from build123d import *

# Parameters (mm, degrees)
F0_W      = 72
F0_H      = 72
F1_DEPTH  = 1.55
F2_W      = 9
F2_H      = 9
F3_DEPTH  = 1.551
F4_R      = 4
F5_W      = 21
F5_H      = 31
F6_DEPTH  = 4
F7_W      = 5.2
F7_H      = 8
F7_W_2    = 0.8
F8_DEPTH  = 2.5
F9_W      = 12.8
F9_H      = 38
F10_DEPTH = 5
F11_W     = 5.5
F11_H     = 11.5
F12_DEPTH = 2.5
F13_R     = 0.75
F14_DEPTH = 4.051
F15_W     = 4.5
F15_H     = 4.5
F16_DEPTH = 3
F17_W     = 7.4
F17_H     = 2.4
F18_DEPTH = 9.3


with BuildPart() as f1:
    # F0 (on Top) → F1 (new body)
    with BuildSketch(Plane.XY):
        with Locations((-36, -36)):
            Rectangle(F0_W, F0_H)
    extrude(amount=-F1_DEPTH)

    # F2 (on face) → F3 (cut, through all)
    with BuildSketch(Plane.XY):
        with Locations((-67.5, -67.5)):
            Rectangle(F2_W, F2_H)
        with Locations((-67.5, -4.5)):
            Rectangle(F2_W, F2_H)
        with Locations((-4.5, -4.5)):
            Rectangle(F2_W, F2_H)
        with Locations((-4.5, -67.5)):
            Rectangle(F2_W, F2_H)
    extrude(amount=-F3_DEPTH, mode=Mode.SUBTRACT)

    # F4
    f4_edges = [f1.edges().sort_by_distance(p)[0] for p in [
        (-9, -63, -0.775),
        (-63, -63, -0.775),
        (-63, -9, -0.775),
        (-9, -9, -0.775),
    ]]
    fillet(f4_edges, radius=F4_R)

    # F5 (on face) → F6 (join)
    with BuildSketch(Plane.XY):
        with Locations((-39, -15.5)):
            Rectangle(F5_W, F5_H)
    extrude(amount=F6_DEPTH)

    # F7 (on face) → F8 (join)
    with BuildSketch(Plane.XY):
        with Locations((-69.4, -20)):
            Rectangle(F7_W, F7_H)
        with Locations((-72.4, -20)):
            Rectangle(F7_W_2, F7_H)
    extrude(amount=F8_DEPTH)

    # F9 (on face) → F10 (join)
    with BuildSketch(Plane.XY):
        with Locations((-5.5, -36)):
            Rectangle(F9_W, F9_H)
    extrude(amount=F10_DEPTH)

    # F11 (on face) → F12 (join)
    with BuildSketch(Plane(origin=(0, 0, -1.55), x_dir=(1, 0, 0), z_dir=(0, 0, -1))):
        with Locations((-67.75, 36.85)):
            Rectangle(F11_W, F11_H)
    extrude(amount=F12_DEPTH)

    # F13 (on face) → F14 (cut, through all)
    with BuildSketch(Plane.XY):
        with Locations((-60, -4)):
            Circle(F13_R)
        with Locations((-12, -4)):
            Circle(F13_R)
        with Locations((-12, -68)):
            Circle(F13_R)
        with Locations((-60, -68)):
            Circle(F13_R)
    extrude(amount=-F14_DEPTH, mode=Mode.SUBTRACT)

    # F15 (on face) → F16 (join)
    with BuildSketch(Plane.XY):
        with Locations((-16.25, -22.05)):
            Rectangle(F15_W, F15_H)
        with Locations((-16.25, -49.95)):
            Rectangle(F15_W, F15_H)
    extrude(amount=F16_DEPTH)

    # F17 (on face) → F18 (join)
    with BuildSketch(Plane.XY):
        with Locations((-59.2, -47.9)):
            Rectangle(F17_W, F17_H)
    extrude(amount=F18_DEPTH)


solid = f1.part
Verification items for the finished model (mm, model axes). A direction names the side the tool comes from. Coordinates: 2 decimals unless noted, no trailing zeros. Loops run counter-clockwise (first coordinate to the right, second up) from the corner with the lowest first, then second, coordinate; pieces in that order, holes last. Notation, with made-up numbers: (14.25, -4.5) -> (36.25, -4.5) arc R15 cw to (36.25, 16.5) -> close; hole circle Ø10 at (19.25, 25). An arc over 180 degrees is marked (long way). Answer as a JSON object with one key per item and string values. Group by question number.
Item 1: Mould release check, pull along X, two halves, no side actions. Record for faces 4 (the flat face through (-16, -52.2, 1)), 5 (the flat face through (-55.5, -48, 5)), 6 (the cylindrical face through (-64.203, -7.859, -0.786)): +X half, -X half, draft (parallel to the pull), parting line (faces both ways), or undercut.
Item 2: Scan lines: probe 1 along X at (y, z) = (-68, -1.2); probe 2 along Y at (x, z) = (-60, -0.9); probe 3 along X at (y, z) = (-30, 0.25). Record each from-to range of solid material in increasing order.
Item 3: Depth check by flat-ended pin: pin 1 (0.7 mm diameter, centred on x = 0.5, y = -41.5, fed in from -Z); pin 2 (0.5 mm diameter, centred on x = -69.5, z = -1, fed in from -Y); pin 3 (1.2 mm diameter, centred on y = -68.5, z = -0.5, fed in from +X). Enter the tip coordinate at first touch or a pass-through.
Item 4: Sectioned sample at C-C on x = -35.5. Record the boundary of the cut face in (y, z), plus the area to 3 significant figures.
Item 5: Sectioned sample at A-A on z = 1.25. Record the boundary of the cut face in (x, y).
Item 6: Tool access check on faces 1 (the flat face through (-70, -16, 1)), 2 (the flat face through (-39, -15, 4)), 3 (the flat face through (-39, -31, 2)). Record the directions out of +Z, -Z, +X, -X, +Y, -Y that give a thin tool (end or side, any length) a straight path to the whole face; none if there is none.
Item 7: Sectioned sample at D-D on y = -22. Record the boundary of the cut face in (x, z), plus the area to 3 significant figures.
Item 8: Sectioned sample at B-B on y = -36.5. Record the boundary of the cut face in (x, z).
Evaluation:
{
 "1": {"face 4": "draft", "face 5": "undercut", "face 6": "-X half"},
 "2": {"probe 1": "x = -63 to -60.75, -59.25 to -12.75, -11.25 to -9", "probe 2": "y = -72 to -68.75, -67.25 to -4.75, -3.25 to 0", "probe 3": "x = -49.5 to -28.5, -11.9 to 0.9"},
 "3": {"pin 1": "stops at z = 0", "pin 2": "stops at y = -63", "pin 3": "stops at x = -9"},
 "4": {"outline": "(-72, -1.55) -> (0, -1.55) -> (0, 4) -> (-31, 4) -> (-31, 0) -> (-72, 0) -> close", "area": "236 mm²"},
 "5": {"outline": "(-72.8, -24) -> (-66.8, -24) -> (-66.8, -16) -> (-72.8, -16) -> close; (-62.9, -49.1) -> (-55.5, -49.1) -> (-55.5, -46.7) -> (-62.9, -46.7) -> close; (-49.5, -31) -> (-28.5, -31) -> (-28.5, 0) -> (-49.5, 0) -> close; (-18.5, -52.2) -> (-14, -52.2) -> (-14, -47.7) -> (-18.5, -47.7) -> close; (-18.5, -24.3) -> (-14, -24.3) -> (-14, -19.8) -> (-18.5, -19.8) -> close; (-11.9, -55) -> (0.9, -55) -> (0.9, -17) -> (-11.9, -17) -> close"},
 "6": {"face 1": "+Z, -X, +Y", "face 2": "+Z, -X, +Y, -Y", "face 3": "+Z, -X, -Y"},
 "7": {"outline": "(-72.8, 0) -> (-72, 0) -> (-72, -1.55) -> (0, -1.55) -> (0, 0) -> (0.9, 0) -> (0.9, 5) -> (-11.9, 5) -> (-11.9, 0) -> (-14, 0) -> (-14, 3) -> (-18.5, 3) -> (-18.5, 0) -> (-28.5, 0) -> (-28.5, 4) -> (-49.5, 4) -> (-49.5, 0) -> (-66.8, 0) -> (-66.8, 2.5) -> (-72.8, 2.5) -> close", "area": "288 mm²"},
 "8": {"outline": "(-72, -1.55) -> (-70.5, -1.55) -> (-70.5, -4.05) -> (-65, -4.05) -> (-65, -1.55) -> (0, -1.55) -> (0, 0) -> (0.9, 0) -> (0.9, 5) -> (-11.9, 5) -> (-11.9, 0) -> (-72, 0) -> close"}
}
